Geometry: see drawing. Coordinates: mm, zero at the bounding-box minimum. A direction names the side the tool comes from. Give positions to 0.01 mm unless a question says otherwise; leave off trailing zeros. Loops run counter-clockwise (first coordinate to the right, second up) from the corner with the lowest first, then second, coordinate; pieces in that order, holes last. Notation, with made-up numbers: M 32.5,27 L 66.5,27 A24 cw 66.5,41 Z; hole C -32.75,15 d7. An arc over 180 degrees is marked long. Use a Markdown table: item, result. Add a question column.
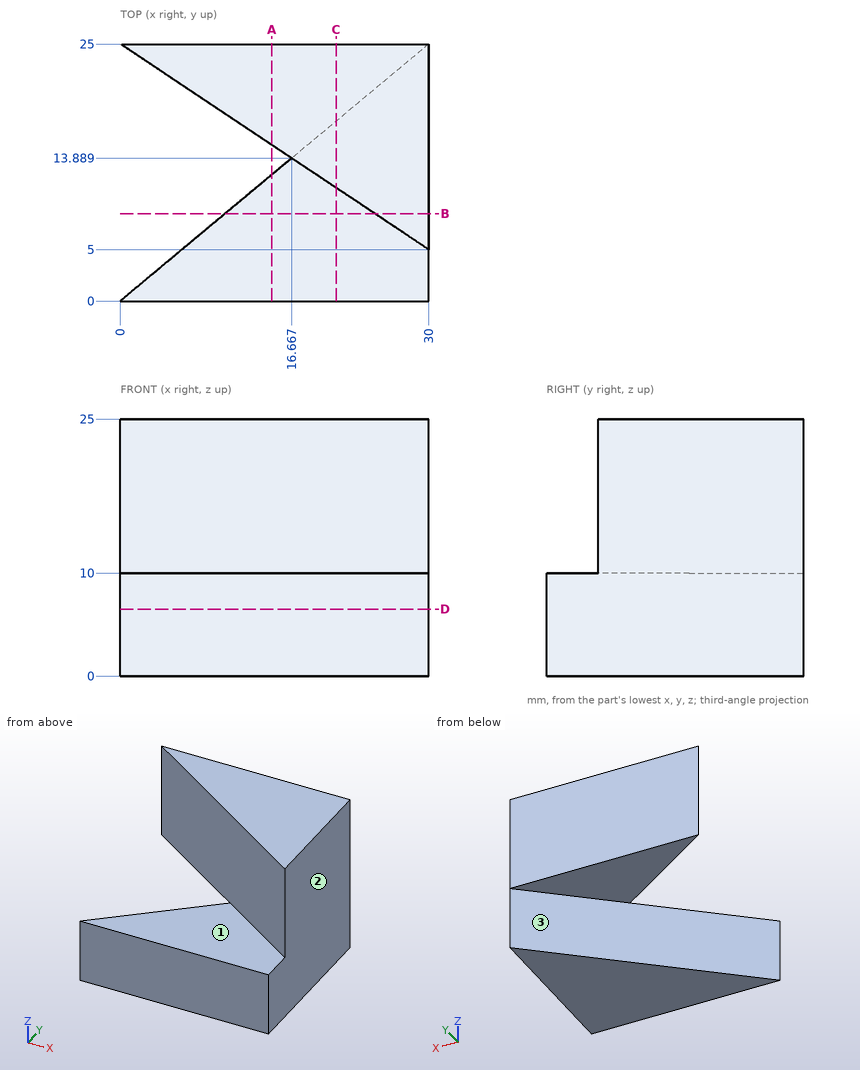
1) Ray query, line 1 (Z direction, x = 15, y = 7.5); line 2 (Z direction, x = 8.25, y = 21); line 3 (X direction, y = 20, z = 8.75). Return the intervals inside material, ascending. Write a range as [from, to].
2) Section query C-C, the plane x = 21. Return the cut outline in (y, z), and give its area (3 significant figures).
3) Contact query for flat-ended pins moving along their axis: P1, Ø2, axis at y = 8.5, z = 6.5, coming from the -X side; P2, Ø12, axis at y = 18.5, z = 13.5, coming from the -X side; P3, Ø5.5, axis at x = 12, y = 20.5, coming from the -Z side. Output: stop coordinate, or through.
4) Section query D-D, the plane z = 6.5. Return the cut outline in (x, y), and give its area (3 significant figures).
5) Section query B-B, the plane y = 8.5. Return the cut outline in (x, z).
6) Reachability of the marked faces 1, 2 and 3 from +Z, -Z, +X, -X, +Y, -Y: full face, straight path, thin tool, end or side. Return the list, or none.
7) Section query A-A, the plane x = 14.75. Return the cut outline in (y, z), and give its area (3 significant figures).
Entries:
| question | item | result |
|---|---|---|
| 1 | line 1 | z = [0, 10] |
| 1 | line 2 | z = [10, 25] |
| 1 | line 3 | x = [24, 30] |
| 2 | outline | M 0,0 L 17.5,0 L 17.5,10 L 25,10 L 25,25 L 11,25 L 11,10 L 0,10 Z |
| 2 | area | 385 mm² |
| 3 | P1 | stops at x = 9 |
| 3 | P2 | stops at x = 0.75 |
| 3 | P3 | stops at z = 10 |
| 4 | outline | M 0,0 L 30,0 L 30,25 Z |
| 4 | area | 375 mm² |
| 5 | outline | M 10.2,0 L 30,0 L 30,25 L 24.75,25 L 24.75,10 L 10.2,10 Z |
| 6 | face 1 | +Z, -X, -Y |
| 6 | face 2 | +Z, -Z, +X, +Y, -Y |
| 6 | face 3 | -Z, -X, +Y |
| 7 | outline | M 0,0 L 12.29,0 L 12.29,10 L 0,10 Z; M 15.17,10 L 25,10 L 25,25 L 15.17,25 Z |
| 7 | area | 270 mm² |
